CAD build for the part. Positions are in the model's coordinates, mm. Face numbers are marked on the shaded views. Round coordinates to 2 decimals unless told otherwise and drop trailing zeros. Write each loop counter-clockwise with the first axis right and the second up, starting at its lowest first coordinate (ties: lowest second). Pieces come first, ordered by that corner, then holes. Notation, with made-up numbers: (40.5, -16.5) - (71.5, -16.5) arc R25 cw to (71.5, 13.5) - close; hole circle Ø2 at (-27.75, -5). An arc over 180 degrees is marked (long way). Answer in a Markdown table with one row per item.
Autodesk Inventor part; units mm, degrees
ref_plane "YZ Plane" through (0, 0, 0) normal (1, 0, 0) x (0, 1, 0)
ref_plane "XZ Plane" through (0, 0, 0) normal (0, 1, 0) x (-1, 0, 0)
ref_plane "XY Plane" through (0, 0, 0) normal (0, 0, 1) x (1, 0, 0)
sketch "Sketch1" plane through (0, 0, 0) normal (0, 0, 1) x (1, 0, 0)
  line L0 (57.5, 0) -> (28.75, -49.7965) construction
  line L1 (28.75, -49.7965) -> (-28.75, -49.7965) construction
  line L2 (-28.75, -49.7965) -> (-57.5, 0) construction
  line L3 (-57.5, 0) -> (-28.75, 49.7965) construction
  line L4 (-28.75, 49.7965) -> (28.75, 49.7965) construction
  line L5 (28.75, 49.7965) -> (57.5, 0) construction
  line L6 (-31.6368, 54.7965) -> (-63.2735, 0) construction
  line L7 (-63.2735, 0) -> (-31.6368, -54.7965) construction
  line L8 (-31.6368, -54.7965) -> (31.6368, -54.7965) construction
  line L9 (31.6368, -54.7965) -> (63.2735, 0) construction
  line L10 (63.2735, 0) -> (31.6368, 54.7965) construction
  line L11 (31.6368, 54.7965) -> (-31.6368, 54.7965) construction
  line L12 (-47.9466, -16.547) -> (-52.2767, -19.047) construction
  line L13 (-45.4466, -20.8771) -> (-49.7767, -23.3771)
  line L14 (-45.4466, -20.8771) -> (-57.5, 0)
  line L15 (-49.7767, -23.3771) -> (-63.2735, 0)
  line L16 (-63.2735, 0) -> (-31.6368, 54.7965)
  line L17 (-31.6368, 54.7965) -> (-28.75, 49.7965)
  line L18 (-28.75, 49.7965) -> (-57.5, 0)
  point P0 (0, 0)
  point P1 (0, 0)
  dimension "d0" = 115
  dimension "d1" = 5
  dimension "d2" = 19.1068
  dimension "d3" = 5
extrude "Extrusion1" add sketch "Sketch1" along normal blind 35
sketch "Sketch2" plane through (-57.5, 0, 35) normal (0.8660254, 0.5, 0) x (0, 0, -1)
  circle A0 centre (17.5, -19.1068) radius 1.5 construction
  line L0 (35, -24.1068) -> (0, -24.1068)
  line L1 (21.5, -19.1068) -> (13.5, -19.1068) construction
  circle A1 centre (21.5, -19.1068) radius 1.5
  circle A2 centre (13.5, -19.1068) radius 1.5
  point P0 (35, -28.75)
  point P1 (17.5, -24.1068)
  dimension "d6" = 3
  dimension "d7" = 5
  dimension "d14" = 8
  dimension "d15" = 3
  dimension "d16" = 3
extrude "Extrusion2" cut sketch "Sketch2" against normal through all
sketch "Sketch3" plane through (0, 0, 35) normal (0, 0, 1) x (1, 0, 0)
  line L0 (-45.4466, -20.8771) -> (-57.5, 0) construction
  line L1 (-57.5, 0) -> (-28.75, 49.7965) construction
  line L2 (-30.4821, 50.7965) -> (-59.8094, 0) construction
  line L3 (-59.8094, 0) -> (-47.1786, -21.8771) construction
  line L4 (-51.5267, -20.346) -> (-53.0267, -17.7479) construction
  line L5 (-48.6966, -15.2479) -> (-47.1966, -17.846) construction
  line L6 (-51.1966, -10.9178) -> (-52.9286, -11.9178)
  line L7 (-51.1966, -10.9178) -> (-57.5, 0)
  line L8 (-57.5, 0) -> (-28.75, 49.7965)
  line L9 (-28.75, 49.7965) -> (-29.9047, 51.7965)
  line L10 (-28.75, 49.7965) -> (-31.6368, 54.7965)
  line L11 (-29.9047, 51.7965) -> (-59.8094, 0)
  line L12 (-59.8094, 0) -> (-52.9286, -11.9178)
  line L13 (-49.7767, -23.3771) -> (-45.4466, -20.8771)
  point P0 (0, 0)
  dimension "d10" = 2
  dimension "d17" = 11.5
extrude "Extrusion3" cut sketch "Sketch3" against normal through all
sketch "Sketch4" plane through (-45.4466, -20.8771, 35) normal (0.8660254, 0.5, 0) x (0, 0, -1)
  line L0 (35, 0) -> (0, 0) construction
  line L1 (35, 11.5) -> (0, 11.5) construction
  line L2 (10, 0) -> (25, 0)
  line L3 (25, 0) -> (25, 11.5)
  line L4 (25, 11.5) -> (10, 11.5)
  line L5 (10, 11.5) -> (10, 0)
  circle A0 centre (13.5, 5) radius 1.5 construction
  line L6 (13.5, 5) -> (21.5, 5) construction
  circle A1 centre (21.5, 5) radius 1.5 construction
  line L7 (10, 11.5) -> (0, 11.5)
  line L8 (0, 11.5) -> (0, 0)
  line L9 (0, 0) -> (10, 0)
  line L10 (10, 0) -> (10, 11.5)
  line L11 (35, 11.5) -> (35, 0)
  line L12 (25, 11.5) -> (35, 11.5)
  line L13 (35, 11.5) -> (35, 0)
  line L14 (35, 0) -> (25, 0)
  line L15 (25, 0) -> (25, 11.5)
  point P0 (35, -4.6432)
  point P1 (17.5, 5)
  point P2 (17.5, 11.5)
  point P3 (17.5, 11.5)
  dimension "d18" = 15
extrude "Extrusion4" cut sketch "Sketch4" against normal blind 2 contours L9 L8 L7 L5 | L3 L12 L11 L14
sketch "Sketch5" plane through (-49.7767, -23.3771, 0) normal (-0.8660254, -0.5, 0) x (0, 0, 1)
  line L0 (0, 0) -> (35, 0)
  line L1 (0, 58.6303) -> (35, 58.6303)
  line L2 (35, 0) -> (28, 0)
  line L3 (28, 0) -> (28, 58.6303)
  line L4 (28, 58.6303) -> (35, 58.6303)
  line L5 (35, 58.6303) -> (35, 0)
  line L6 (0, 0) -> (7, 0)
  line L7 (7, 0) -> (7, 58.6303)
  line L8 (7, 58.6303) -> (0, 58.6303)
  line L9 (0, 58.6303) -> (0, 0)
  point P0 (0, -4.6432)
  dimension "d21" = 7
  dimension "d24" = 7
extrude "Extrusion5" cut sketch "Sketch5" against normal through all contours L9 L1 L7 L0
properties part number "TA09" material "ABS Plastic"
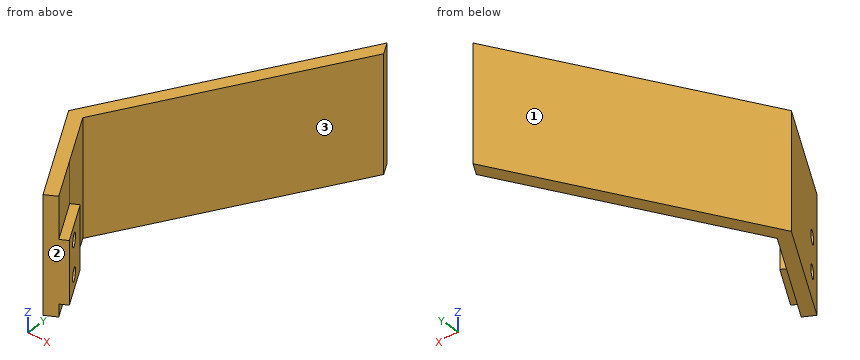
Q1. Saw through at C-C on z = 16. List the corners of the cut face in (x, y).
Computed:
| item | result |
|---|---|
| outline | (-63.27, 0) - (-49.78, -23.38) - (-45.45, -20.88) - (-51.2, -10.92) - (-52.93, -11.92) - (-59.81, 0) - (-29.9, 51.8) - (-31.64, 54.8) - close |
Q2. Flat gauge pins, fed straight in: pin 1 (8 mm diameter, centred on x = -58.5, z = 29, fed in from +Y); pin 2 (12 mm diameter, centred on y = 3, z = 31, fed in from +X); pin 3 (2 mm diameter, centred on y = 30, z = 18.5, fed in from -X). Where does each tip first touch, or does it go through?
Computed:
| item | result |
|---|---|
| pin 1 | stops at y = 15.2 |
| pin 2 | stops at x = -54.61 |
| pin 3 | stops at x = -46.53 |
Q3. Drill centre lines: line 1 (Y direction, x = -50, z = 22); line 2 (Y direction, x = -57.5, z = 10.75); line 3 (Y direction, x = -52, z = 31.5). Where is each one in solid material? Low to high.
Computed:
| item | result |
|---|---|
| line 1 | y = -22.99 to -19.37, -16.1 to -12.99, 16.99 to 22.99 |
| line 2 | y = -10 to -4, 4 to 10 |
| line 3 | y = -19.53 to -13.53, 13.53 to 19.53 |
Q4. Saw through at A-A on z = 21.25. List the corners of the cut face in (x, y).
Computed:
| item | result |
|---|---|
| outline | (-63.27, 0) - (-53.02, -17.77) - (-48.69, -15.27) - (-51.2, -10.92) - (-52.93, -11.92) - (-59.81, 0) - (-29.9, 51.8) - (-31.64, 54.8) - close; (-51.54, -20.33) - (-49.78, -23.38) - (-45.45, -20.88) - (-47.21, -17.83) - close |
Q5. Saw through at D-D on y = -13. List the corners of the cut face in (x, z), then the cut area to 3 significant figures.
Computed:
| item | result |
|---|---|
| outline | (-55.77, 7) - (-52.31, 7) - (-52.31, 10) - (-49.99, 10) - (-49.99, 25) - (-52.31, 25) - (-52.31, 35) - (-55.77, 35) - close |
| area | 132 mm2 |
Q6. Pull direction Y, two halves, no side cores. Call the marked faces 1, 2 and 3: released by +Y, released by -Y, zero draft, split by the parting line, or undercut.
Computed:
| item | result |
|---|---|
| face 1 | released by +Y |
| face 2 | released by -Y |
| face 3 | undercut |
Q7. Saw through at B-B on x = -55.5. List the corners of the cut face in (y, z).
Computed:
| item | result |
|---|---|
| outline | (-13.46, 7) - (-7.46, 7) - (-7.46, 35) - (-13.46, 35) - close; (7.46, 7) - (13.46, 7) - (13.46, 35) - (7.46, 35) - close |
